Part model, mm, in its own coordinate system. A direction names the side the tool comes from. Give positions to 0.01 mm unless a question says otherwise; leave off trailing zeros. Order: outer loops, then holes, each group sorted by start corner. A loop starts at its lowest first (then second) coordinate and runs counter-clockwise, first axis right, second up. Notation, with made-up numbers: (72, -30.75) -> (119, -30.75) arc R18 ccw to (119, -0.75) -> close; hole circle Ø9 at (63.5, 77.25). An arc over 180 degrees is marked (long way). Write item = value, one per line. Start each with the question number.
(1) Saw through at B-B, the plane x = 52. List the corners of the cut face in (y, z), then the cut area to 3 significant figures.
(2) Saw through at A-A, the plane y = 63.5. List the corners of the cut face in (x, z).
(3) Flat gauge pins, fed straight in: pin 1 (8 mm diameter, centred on y = -129, z = 10, fed in from +X); pin 2 (4 mm diameter, centred on y = 118.5, z = 14, fed in from +X); pin 3 (1.5 mm diameter, centred on x = 0.5, z = 13.5, fed in from -Y); pin 4 (12 mm diameter, centred on x = -2, y = -12.5, fed in from -Z). Where does each tip first touch, or does it go through?
(4) Probe line 1 along Y through (x, z) = (21, 12); line 2 along Y through (x, z) = (-3, 14.5); line 3 along X through (y, z) = (62.5, 2.5). List the from-to ranges inside material, lowest first. Write a range as from..to.
(5) Two-plate mould, pull along Z, no slides. Class faces 4 (the cylindrical face through (68.532, -85.966, 14.989)), 5 (the flat face through (-50, -146.667, 13)), 6 (the cylindrical face through (-65.484, 107.801, 12.878)): pulls with the +Z half, pulls with the -Z half, needs draft (parallel to the pull), parting line crosses it, or undercut.
(6) Which spindle directions (+Z, -Z, +X, -X, +Y, -Y) get a long thin tool onto all of the face, cutting with end or side? Do faces 1 (the flat face through (8.271, -160, 13)), 2 (the flat face through (-5, -26, 0)), 3 (the flat face through (64, -129, 17.78)). Say none if no direction does.
from build123d import *

# Parameters (mm, degrees)
F0_W      = 140.7454609871
F0_H      = 288.360491395
F1_DEPTH  = 25.4
F4_DEPTH  = 25.4
F6_W      = 16.9358227252
F6_H      = 4.5118425041
F7_DEPTH  = 3.81
F8_W      = 13.9597124967
F8_H      = 10.16
F9_DEPTH  = 6.35
F8_R      = 7.62
F11_DEPTH = 3.81
F5_W      = 24.153170515
F5_H      = 5.08
F12_DEPTH = 25.4
F5_R      = 4.5118428767
F13_DEPTH = 25.4


with BuildPart() as f1:
    # F0 (on Top) → F1 (new body)
    with BuildSketch(Plane.XY):
        with Locations((-3.7190392613, -27.8867259622)):
            Rectangle(F0_W, F0_H)
    extrude(amount=F1_DEPTH)

    # F2 (on face) → F4 (cut)
    with BuildSketch(Plane.XY.offset(25.4)):
        with BuildLine():
            ThreePointArc((66.6536912322, -144.3410718666), (57.604458326, -164.0297686766), (37.4814176394, -172.0669716597))
            Line((37.4814176394, -172.0669716597), (66.6536912322, -172.0669716597))
            Line((66.6536912322, -172.0669716597), (66.6536912322, -144.3410718666))
        make_face()
        with BuildLine():
            Line((-74.0917697549, -172.0669716597), (-45.0917528756, -172.0669716597))
            ThreePointArc((-45.0917528756, -172.0669716597), (-64.4708824202, -164.7127131958), (-74.0917697549, -146.3531296941))
            Line((-74.0917697549, -146.3531296941), (-74.0917697549, -172.0669716597))
        make_face()
        with BuildLine():
            ThreePointArc((41.1493752002, 116.2935197353), (58.7544153268, 107.3576281035), (66.6536912322, 89.2637330754))
            Line((66.6536912322, 89.2637330754), (66.6536912322, 116.2935197353))
            Line((66.6536912322, 116.2935197353), (41.1493752002, 116.2935197353))
        make_face()
        with BuildLine():
            Line((-74.0917697549, 116.2935197353), (-74.0917697549, 87.8933618236))
            ThreePointArc((-74.0917697549, 87.8933618236), (-65.2592523832, 108.0224737135), (-44.8929982774, 116.2935197353))
            Line((-44.8929982774, 116.2935197353), (-74.0917697549, 116.2935197353))
        make_face()
    extrude(amount=-F4_DEPTH, mode=Mode.SUBTRACT)

    # F6 (on face) → F7 (join)
    with BuildSketch(Plane(origin=(0, 116.2935197353, 0), x_dir=(-1, 0, 0), z_dir=(0, 1, 0))):
        with Locations((-32.6814638376, 13.2347373292)):
            Rectangle(F6_W, F6_H)
    extrude(amount=F7_DEPTH)

    # F8 (on face) → F9 (cut)
    with BuildSketch(Plane.YZ.offset(66.6536912322)):
        with Locations((-128.4659260378, 12.7)):
            Rectangle(F8_W, F8_H)
    extrude(amount=-F9_DEPTH, mode=Mode.SUBTRACT)

    # F8 (on face) → F11 (join)
    with BuildSketch(Plane.YZ.offset(66.6536912322)):
        with Locations((-109.8529842751, 12.7)):
            Circle(F8_R)
        with Locations((-93.2342812741, 12.7)):
            Circle(F8_R)
    extrude(amount=F11_DEPTH)

    # F5 (on face) → F12 (cut)
    with BuildSketch(Plane.XZ.offset(172.0669716597)):
        with Locations((-3.8051676181, 12.7)):
            Rectangle(F5_W, F5_H)
    extrude(amount=-F12_DEPTH, mode=Mode.SUBTRACT)

    # F5 (on face) → F13 (cut)
    with BuildSketch(Plane.XZ.offset(172.0669716597)):
        with Locations((-50.3822378814, 13.0843427032)):
            Circle(F5_R)
    extrude(amount=-F13_DEPTH, mode=Mode.SUBTRACT)


solid = f1.part
Results list:
q1.outline = (-168.2, 0) -> (112.67, 0) -> (112.67, 25.4) -> (-168.2, 25.4) -> close
q1.area = 7,130 mm^2
q2.outline = (-74.09, 0) -> (66.65, 0) -> (66.65, 25.4) -> (-74.09, 25.4) -> close
q3.pin_1 = 66.65
q3.pin_2 = 41.15
q3.pin_3 = -146.67
q3.pin_4 = 0
q4.line_1 = -172.07..116.29
q4.line_2 = -146.67..116.29
q4.line_3 = -74.09..66.65
q5.face_4 = parting line crosses it
q5.face_5 = undercut
q5.face_6 = needs draft
q6.face_1 = -Y
q6.face_2 = -Z, +X, -X, +Y, -Y
q6.face_3 = +X
